The model under review builds one solid part; all positions refer to its coordinate system, in mm. Face numbers are marked on the shaded views. A direction names the side the tool comes from. Coordinates: 2 decimals unless noted, no trailing zeros. Write each loop counter-clockwise with the first axis right and the second up, starting at its lowest first coordinate (ties: lowest second). Pieces come first, ordered by that corner, then holes.
1) Add section C-C, the plane x = 0. State the section outline as (y, z) points.
2) For line 1 (Y direction, x = 1.5, z = 33); line 2 (Y direction, x = 0.5, z = 25); line 3 (Y direction, x = 0.25, z = -5), list the stretches that pass through material, from the lowest coordinate up.
3) Machinability: for the marked faces 1, 2 and 3, which of the approach directions +Z, -Z, +X, -X, +Y, -Y give a long, thin tool a straight path to every point of the face, cutting with its end or side? Answer none if there is none.
4) For P1, Ø3.5, axis at x = -1, z = 35, coming from the +Y side; P2, Ø3, axis at y = -3.5, z = 13, coming from the -X side; P3, Ø1.5, axis at y = 0, z = 24.5, coming from the -X side, all flat-tipped, find the tip position at first contact; note any pin that passes through.
5) Add section A-A, the plane y = 0. State the section outline as (x, z) points.
6) Add section B-B, the plane z = 33. State the section outline as (x, y) points.
7) Add section D-D, the plane y = -3. State the section outline as (x, z) points.
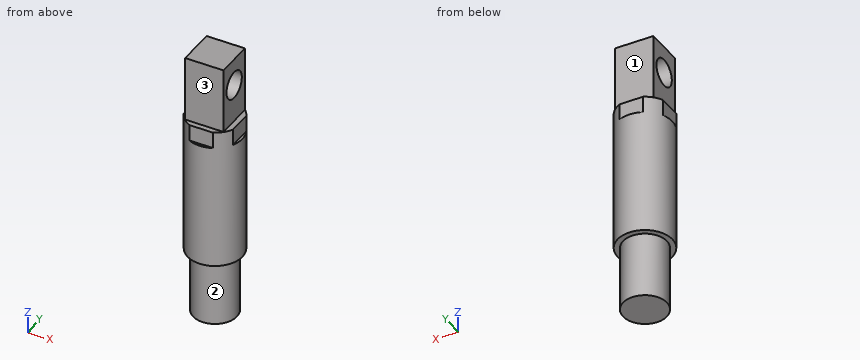
from build123d import *

# Parameters (mm, degrees)
ESQUISSE1_R             = 5
BOSS_EXTRU_2_DEPTH      = 70
ESQUISSE2_R             = 3.5
BOSS_EXTRU_3_DEPTH      = 12
ESQUISSE4_R             = 15
BOSS_EXTRU_5_DEPTH      = 5
ESQUISSE5_R             = 3.5
BOSS_EXTRU_6_DEPTH      = 12
ENL_V_MAT_EXTRU_1_DEPTH = 12
ESQUISSE7_R             = 15
ENL_V_MAT_EXTRU_2_DEPTH = 47
ESQUISSE8_W             = 9
ESQUISSE8_H             = 9
BOSS_EXTRU_7_DEPTH      = 5
ESQUISSE9_W             = 10
ESQUISSE9_H             = 10
ESQUISSE9_W_2           = 9
ESQUISSE9_H_2           = 9
ENL_V_MAT_EXTRU_3_DEPTH = 12
ESQUISSE10_W            = 9
ESQUISSE10_H            = 9
BOSS_EXTRU_8_DEPTH      = 7
ESQUISSE11_W            = 9
ESQUISSE11_H            = 9
ENL_V_MAT_EXTRU_4_DEPTH = 4
ESQUISSE13_W            = 9
ESQUISSE13_H            = 9
BOSS_EXTRU_9_DEPTH      = 12
ESQUISSE14_W            = 9
ESQUISSE14_H            = 9
ESQUISSE14_W_2          = 7
ESQUISSE14_H_2          = 7
ENL_V_MAT_EXTRU_5_DEPTH = 12
ESQUISSE15_R            = 2.5
ENL_V_MAT_EXTRU_6_DEPTH = 12
ESQUISSE16_R            = 4
BOSS_EXTRU_10_DEPTH     = 12


with BuildPart() as part:
    # Esquisse1 → Boss.-Extru.2 (new body)
    with BuildSketch(Plane.XY):
        Circle(ESQUISSE1_R)
    extrude(amount=BOSS_EXTRU_2_DEPTH)

    # Esquisse2 → Boss.-Extru.3 (add)
    with BuildSketch(Plane(origin=(0, 0, 0), x_dir=(-1, 0, 0), z_dir=(0, 0, -1))):
        Circle(ESQUISSE2_R)
    extrude(amount=BOSS_EXTRU_3_DEPTH)

    # Esquisse4 → Boss.-Extru.5 (add)
    with BuildSketch(Plane.XY.offset(70)):
        Circle(ESQUISSE4_R)
    extrude(amount=-BOSS_EXTRU_5_DEPTH)

    # Esquisse5 → Boss.-Extru.6 (add)
    with BuildSketch(Plane.XY.offset(70)):
        Circle(ESQUISSE5_R)
    extrude(amount=BOSS_EXTRU_6_DEPTH)

    # Esquisse6 → Enlèv. mat.-Extru.1 (cut)
    with BuildSketch(Plane.XY.offset(70)):
        with BuildLine():
            Line((-6.262893089, 8.172072336), (-7.499435292, 12.990707074))
            ThreePointArc((-7.499435292, 12.990707074), (-9.123657799, 11.90625333), (-10.593218546, 10.619968024))
            Line((-10.593218546, 10.619968024), (-6.262893089, 8.172072336))
        make_face()
        with BuildLine():
            Line((-8.152402023, 6.270263162), (-10.606442664, 10.606760769))
            ThreePointArc((-10.606442664, 10.606760769), (-11.894621233, 9.138817524), (-12.981158937, 7.515950549))
            Line((-12.981158937, 7.515950549), (-8.152402023, 6.270263162))
        make_face()
        with BuildLine():
            Line((-9.499942261, 3.951679007), (-12.981158937, 7.515950549))
            ThreePointArc((-12.981158937, 7.515950549), (-13.849269023, 5.761748652), (-14.481582106, 3.909447494))
            Line((-14.481582106, 3.909447494), (-9.499942261, 3.951679007))
        make_face()
        with BuildLine():
            Line((-10.188028074, 1.356459322), (-14.486441985, 3.891400598))
            ThreePointArc((-14.486441985, 3.891400598), (-14.869805294, 1.972027008), (-14.999987869, 0.0190767))
            Line((-14.999987869, 0.0190767), (-10.188028074, 1.356459322))
        make_face()
        with BuildLine():
            ThreePointArc((-14.999987869, -0.0190767), (-14.869805294, -1.972027008), (-14.486441985, -3.891400598))
            Line((-14.486441985, -3.891400598), (-10.188028074, -1.356459322))
            Line((-10.188028074, -1.356459322), (-14.999987869, -0.0190767))
        make_face()
        with BuildLine():
            Line((-9.499942261, -3.951679007), (-14.481582106, -3.909447494))
            ThreePointArc((-14.481582106, -3.909447494), (-13.849269023, -5.761748652), (-12.981158937, -7.515950549))
            Line((-12.981158937, -7.515950549), (-9.499942261, -3.951679007))
        make_face()
        with BuildLine():
            Line((-8.152402023, -6.270263162), (-12.981158937, -7.515950549))
            ThreePointArc((-12.981158937, -7.515950549), (-11.894621233, -9.138817524), (-10.606442664, -10.606760769))
            Line((-10.606442664, -10.606760769), (-8.152402023, -6.270263162))
        make_face()
        with BuildLine():
            Line((-6.262893089, -8.172072336), (-10.593218546, -10.619968024))
            ThreePointArc((-10.593218546, -10.619968024), (-9.123657799, -11.90625333), (-7.499435292, -12.990707074))
            Line((-7.499435292, -12.990707074), (-6.262893089, -8.172072336))
        make_face()
        with BuildLine():
            Line((-3.939593974, -9.504960245), (-7.499435292, -12.990707074))
            ThreePointArc((-7.499435292, -12.990707074), (-5.744130769, -13.8565855), (-3.891026946, -14.486542352))
            Line((-3.891026946, -14.486542352), (-3.939593974, -9.504960245))
        make_face()
        with BuildLine():
            Line((-1.343501295, -10.189744953), (-3.872973884, -14.491379275))
            ThreePointArc((-3.872973884, -14.491379275), (-1.953114292, -14.872301253), (0, -15))
            Line((0, -15), (-1.343501295, -10.189744953))
        make_face()
        with BuildLine():
            ThreePointArc((0, -15), (1.953114292, -14.872301253), (3.872973884, -14.491379275))
            Line((3.872973884, -14.491379275), (1.343501295, -10.189744953))
            Line((1.343501295, -10.189744953), (0, -15))
        make_face()
        with BuildLine():
            ThreePointArc((3.891026946, -14.486542352), (5.744130769, -13.8565855), (7.499435292, -12.990707074))
            Line((7.499435292, -12.990707074), (3.939593974, -9.504960245))
            Line((3.939593974, -9.504960245), (3.891026946, -14.486542352))
        make_face()
        with BuildLine():
            ThreePointArc((7.499435292, -12.990707074), (9.123657799, -11.90625333), (10.593218546, -10.619968024))
            Line((10.593218546, -10.619968024), (6.262893089, -8.172072336))
            Line((6.262893089, -8.172072336), (7.499435292, -12.990707074))
        make_face()
        with BuildLine():
            ThreePointArc((10.606442664, -10.606760769), (11.894621233, -9.138817524), (12.981158937, -7.515950549))
            Line((12.981158937, -7.515950549), (8.152402023, -6.270263162))
            Line((8.152402023, -6.270263162), (10.606442664, -10.606760769))
        make_face()
        with BuildLine():
            ThreePointArc((12.981158937, -7.515950549), (13.849269023, -5.761748652), (14.481582106, -3.909447494))
            Line((14.481582106, -3.909447494), (9.499942261, -3.951679007))
            Line((9.499942261, -3.951679007), (12.981158937, -7.515950549))
        make_face()
        with BuildLine():
            ThreePointArc((15, 0), (14.999996967, 0.009538352), (14.999987869, 0.0190767))
            Line((14.999987869, 0.0190767), (10.159352957, -1.339548494))
            Line((10.159352957, -1.339548494), (14.486441985, -3.891400598))
            ThreePointArc((14.486441985, -3.891400598), (14.87105628, -1.962571047), (15, 0))
        make_face()
        with BuildLine():
            ThreePointArc((14.999987869, 0.0190767), (14.869805294, 1.972027008), (14.486441985, 3.891400598))
            Line((14.486441985, 3.891400598), (10.188028074, 1.356459322))
            Line((10.188028074, 1.356459322), (14.999987869, 0.0190767))
        make_face()
        with BuildLine():
            ThreePointArc((14.481582106, 3.909447494), (13.849269023, 5.761748652), (12.981158937, 7.515950549))
            Line((12.981158937, 7.515950549), (9.499942261, 3.951679007))
            Line((9.499942261, 3.951679007), (14.481582106, 3.909447494))
        make_face()
        with BuildLine():
            ThreePointArc((12.981158937, 7.515950549), (11.894621233, 9.138817524), (10.606442664, 10.606760769))
            Line((10.606442664, 10.606760769), (8.152402023, 6.270263162))
            Line((8.152402023, 6.270263162), (12.981158937, 7.515950549))
        make_face()
        with BuildLine():
            ThreePointArc((10.593218546, 10.619968024), (9.123657799, 11.90625333), (7.499435292, 12.990707074))
            Line((7.499435292, 12.990707074), (6.262893089, 8.172072336))
            Line((6.262893089, 8.172072336), (10.593218546, 10.619968024))
        make_face()
        with BuildLine():
            ThreePointArc((7.499435292, 12.990707074), (5.744130769, 13.8565855), (3.891026946, 14.486542352))
            Line((3.891026946, 14.486542352), (3.939593974, 9.504960245))
            Line((3.939593974, 9.504960245), (7.499435292, 12.990707074))
        make_face()
        with BuildLine():
            ThreePointArc((3.872973884, 14.491379275), (1.953114292, 14.872301253), (0, 15))
            Line((0, 15), (1.343501295, 10.189744953))
            Line((1.343501295, 10.189744953), (3.872973884, 14.491379275))
        make_face()
        with BuildLine():
            Line((-1.343501295, 10.189744953), (0, 15))
            ThreePointArc((0, 15), (-1.953114292, 14.872301253), (-3.872973884, 14.491379275))
            Line((-3.872973884, 14.491379275), (-1.343501295, 10.189744953))
        make_face()
        with BuildLine():
            Line((-3.939593974, 9.504960245), (-3.891026946, 14.486542352))
            ThreePointArc((-3.891026946, 14.486542352), (-5.744130769, 13.8565855), (-7.499435292, 12.990707074))
            Line((-7.499435292, 12.990707074), (-3.939593974, 9.504960245))
        make_face()
    extrude(amount=-ENL_V_MAT_EXTRU_1_DEPTH, mode=Mode.SUBTRACT)

    # Esquisse7 → Enlèv. mat.-Extru.2 (cut)
    with BuildSketch(Plane.XY.offset(82)):
        Circle(ESQUISSE7_R)
    extrude(amount=-ENL_V_MAT_EXTRU_2_DEPTH, mode=Mode.SUBTRACT)

    # Esquisse8 → Boss.-Extru.7 (add)
    with BuildSketch(Plane.XY.offset(35)):
        Rectangle(ESQUISSE8_W, ESQUISSE8_H)
    extrude(amount=-BOSS_EXTRU_7_DEPTH)

    # Esquisse9 → Enlèv. mat.-Extru.3 (cut)
    with BuildSketch(Plane.XY.offset(35)):
        Rectangle(ESQUISSE9_W, ESQUISSE9_H)
        Rectangle(ESQUISSE9_W_2, ESQUISSE9_H_2, mode=Mode.SUBTRACT)
    extrude(amount=-ENL_V_MAT_EXTRU_3_DEPTH, mode=Mode.SUBTRACT)

    # Esquisse10 → Boss.-Extru.8 (add)
    with BuildSketch(Plane.XY.offset(35)):
        Rectangle(ESQUISSE10_W, ESQUISSE10_H)
    extrude(amount=BOSS_EXTRU_8_DEPTH)

    # Esquisse11 → Enlèv. mat.-Extru.4 (cut)
    with BuildSketch(Plane.XY.offset(42)):
        Rectangle(ESQUISSE11_W, ESQUISSE11_H)
    extrude(amount=-ENL_V_MAT_EXTRU_4_DEPTH, mode=Mode.SUBTRACT)

    # Esquisse13 → Boss.-Extru.9 (add)
    with BuildSketch(Plane.XY.offset(38)):
        Rectangle(ESQUISSE13_W, ESQUISSE13_H)
    extrude(amount=-BOSS_EXTRU_9_DEPTH)

    # Esquisse14 → Enlèv. mat.-Extru.5 (cut)
    with BuildSketch(Plane.XY.offset(38)):
        Rectangle(ESQUISSE14_W, ESQUISSE14_H)
        Rectangle(ESQUISSE14_W_2, ESQUISSE14_H_2, mode=Mode.SUBTRACT)
    extrude(amount=-ENL_V_MAT_EXTRU_5_DEPTH, mode=Mode.SUBTRACT)

    # Esquisse15 → Enlèv. mat.-Extru.6 (cut)
    with BuildSketch(Plane(origin=(3.5, 0, 0), x_dir=(0, 0, -1), z_dir=(1, 0, 0))):
        with Locations((-33, 0)):
            Circle(ESQUISSE15_R)
    extrude(amount=-ENL_V_MAT_EXTRU_6_DEPTH, mode=Mode.SUBTRACT)

    # Esquisse16 → Boss.-Extru.10 (add)
    with BuildSketch(Plane(origin=(0, 0, -12), x_dir=(-1, 0, 0), z_dir=(0, 0, -1))):
        Circle(ESQUISSE16_R)
    extrude(amount=-BOSS_EXTRU_10_DEPTH)


solid = part.part
Geometry results:
1. outline: (-5, 0) - (-4, 0) - (-4, -12) - (4, -12) - (4, 0) - (5, 0) - (5, 23) - (4.5, 23) - (4.5, 26) - (3.5, 26) - (3.5, 38) - (-3.5, 38) - (-3.5, 26) - (-4.5, 26) - (-4.5, 23) - (-5, 23) - close; hole circle Ø5 at (0, 33)
2. line 1: y = -3.5 to -2.5, 2.5 to 3.5
2. line 2: y = -4.5 to 4.5
2. line 3: y = -3.99 to 3.99
3. face 1: +Z, +X, -X, +Y
3. face 2: -Z
3. face 3: +Z, +X, -X, -Y
4. P1: stops at y = 3.5
4. P2: stops at x = -4.58
4. P3: stops at x = -4.5
5. outline: (-5, 0) - (-4, 0) - (-4, -12) - (4, -12) - (4, 0) - (5, 0) - (5, 23) - (4.5, 23) - (4.5, 26) - (3.5, 26) - (3.5, 30.5) - (-3.5, 30.5) - (-3.5, 26) - (-4.5, 26) - (-4.5, 23) - (-5, 23) - close; (-3.5, 35.5) - (3.5, 35.5) - (3.5, 38) - (-3.5, 38) - close
6. outline: (-3.5, -3.5) - (3.5, -3.5) - (3.5, -2.5) - (-3.5, -2.5) - close; (-3.5, 2.5) - (3.5, 2.5) - (3.5, 3.5) - (-3.5, 3.5) - close
7. outline: (-4, 0) - (-2.65, 0) - (-2.65, -12) - (2.65, -12) - (2.65, 0) - (4, 0) - (4, 26) - (3.5, 26) - (3.5, 38) - (-3.5, 38) - (-3.5, 26) - (-4, 26) - close
